```python
from build123d import *

# Parameters (mm, degrees)
SKETCH_2_W                   = 295
SKETCH_2_H                   = 12
EXTRUDE_1_DEPTH              = 25
PATTERN_LINEAR_1_COUNT       = 12
PATTERN_LINEAR_1_PITCH       = 25
HOLE_WIZARD_M4_1_D           = 4.5
HOLE_WIZARD_M4_1_CBORE_D     = 8
HOLE_WIZARD_M4_1_CBORE_DEPTH = 4.5
PATTERN_LINEAR_2_COUNT       = 11
PATTERN_LINEAR_2_PITCH       = 25


with BuildPart() as part:
    # 草图2 → 拉伸1 (new body)
    with BuildSketch(Plane(origin=(0, 0, 0), x_dir=(1, 0, 0), z_dir=(0, 1, 0))):
        with Locations((147.5, 0)):
            Rectangle(SKETCH_2_W, SKETCH_2_H)
    extrude(amount=EXTRUDE_1_DEPTH)

    # 草图4 → M3 螺纹孔1 (revolve, cut)
    with BuildSketch(Plane(origin=(10, 25, 0), x_dir=(0, 0, 1), z_dir=(1, 0, 0))):
        Polygon((0, 0), (0, 8.251075774), (1.25, 7.5), (1.25, 0), align=None)
    hole_wizard_m3_1 = revolve(axis=Axis((10, 31.35, 0), (0, -1, 0)), mode=Mode.SUBTRACT)

    # 阵列(线性)1: M3 螺纹孔1 ×12
    with Locations(*[(i * PATTERN_LINEAR_1_PITCH, 0, 0) for i in range(1, PATTERN_LINEAR_1_COUNT)]):
        add(hole_wizard_m3_1, mode=Mode.SUBTRACT)

    # M4 六角凹头螺钉的柱形沉头孔1 (through all)
    with Locations(Plane(origin=(262.846314279, 25, 7.813441093), x_dir=(-1, 0, 0), z_dir=(0, 1, 0))):
        with Locations((240.346314279, -7.813441093)):
            hole_wizard_m4_1 = CounterBoreHole(HOLE_WIZARD_M4_1_D / 2, HOLE_WIZARD_M4_1_CBORE_D / 2, HOLE_WIZARD_M4_1_CBORE_DEPTH)

    # 阵列(线性)2: M4 六角凹头螺钉的柱形沉头孔1 ×11
    with Locations(*[(i * PATTERN_LINEAR_2_PITCH, 0, 0) for i in range(1, PATTERN_LINEAR_2_COUNT)]):
        add(hole_wizard_m4_1, mode=Mode.SUBTRACT)


solid = part.part
```
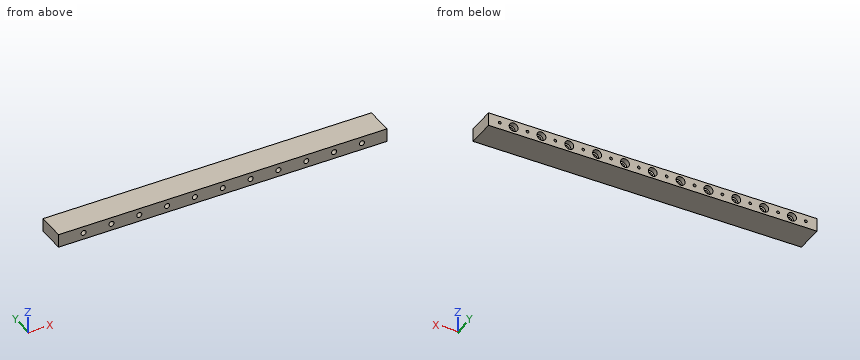
Here's how the part is built. I have some questions about the finished solid (model axes, mm). Coordinates: 2 decimals unless noted, no trailing zeros. One line per item, written item: value.
1) I need wall thicknesses on line 1 along Z through (x, y) = (147.5, 22.3); line 2 along Z through (x, y) = (97.5, 11.25); line 3 along Y through (x, z) = (211, 0.25). Which ranges of each line are inside material? Lowest first, please.
Model answer:
line 1: z = -6 to -4, 4 to 6
line 2: z = -6 to -2.25, 2.25 to 6
line 3: y = 0 to 17.37
2) I'm going to push flat-ended pins straight in: P1, Ø7, axis at x = 47.5, z = 0, coming from the +Y side; P2, Ø1.5, axis at x = 135, z = 0, coming from the +Y side. Where does each tip first touch, or does it pass through?
Model answer:
P1: stops at y = 20.5
P2: stops at y = 17.2
3) Suppose I cut it at A-A on y = 5.5. State how many separate pieces and enclosed holes the cut face has, and give its area (3 significant figures).
Model answer:
separate pieces: 1
enclosed holes: 11
area: 3,370 mm²
